Design review of the part shown in the three views and the two pictorial views. Dimensions are in mm from the part's minimum x, y and z. Round coordinates to 2 decimals unless told otherwise and drop trailing zeros. Loops run counter-clockwise (first coordinate to the right, second up) from the corner with the lowest first, then second, coordinate; pieces in that order, holes last. Notation, with made-up numbers: M 82,17.5 L 136,17.5 A24 ccw 136,52.5 Z; hole C 20,18 d10. An arc over 180 degrees is marked long. Answer as CSV lines item,"result". Start each with the question number.
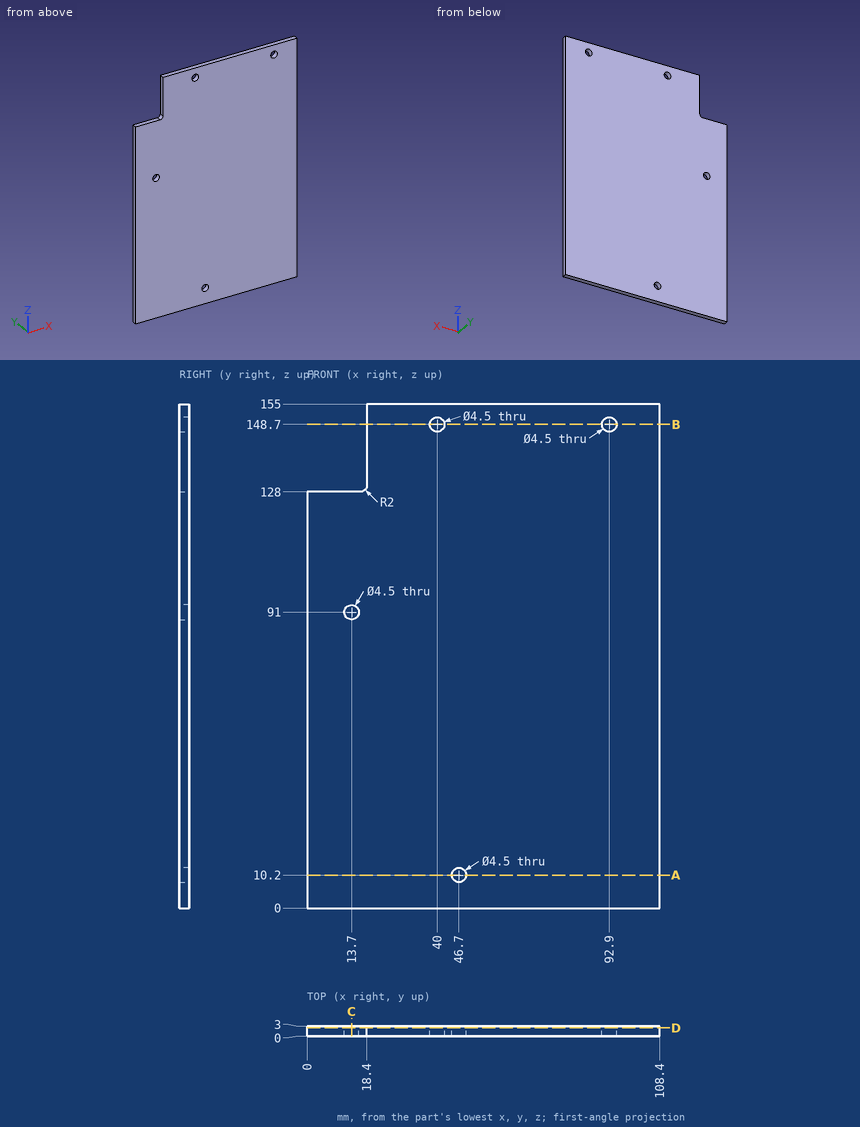
Item 1: Insertion check: pin 1 Ø0.9 at (x, y) = (10, 1) entering from +Z. The pin has a flat end and moves straight along its axis. Give the tip position at first contact, or say it passes through.
Item 2: To check wall thickness, follow line 1 (X direction, y = 1.75, z = 10.2); line 2 (Z direction, x = 15, y = 2.7); line 3 (X direction, y = 1.3, z = 93). State the ranges of each line that lie inside material, in increasing order.
Item 3: Consider section B-B, the plane z = 148.7. Write out the cut boundary in (x, y).
Item 4: Consider section D-D, the plane y = 2.5. Write out the cut boundary in (x, z).
Item 5: Consider section C-C, the plane x = 13.7. Write out the cut boundary in (y, z).
Item 6: Consider section A-A, the plane z = 10.2. Write out the cut boundary in (x, y), then the cut area to 3 significant figures.
Found:
1,pin 1,"stops at z = 128"
2,line 1,"x = 0 to 44.45, 48.95 to 108.4"
2,line 2,"z = 0 to 89.16, 92.84 to 128"
2,line 3,"x = 0 to 12.67, 14.73 to 108.4"
3,outline,"M 18.4,0 L 37.75,0 L 37.75,3 L 18.4,3 Z; M 42.25,0 L 90.65,0 L 90.65,3 L 42.25,3 Z; M 95.15,0 L 108.4,0 L 108.4,3 L 95.15,3 Z"
4,outline,"M 0,0 L 108.4,0 L 108.4,155 L 18.4,155 L 18.4,130 A2 cw 16.4,128 L 0,128 Z; hole C 13.7,91 d4.5; hole C 40,148.7 d4.5; hole C 46.7,10.2 d4.5; hole C 92.9,148.7 d4.5"
5,outline,"M 0,0 L 3,0 L 3,88.75 L 0,88.75 Z; M 0,93.25 L 3,93.25 L 3,128 L 0,128 Z"
6,outline,"M 0,0 L 44.45,0 L 44.45,3 L 0,3 Z; M 48.95,0 L 108.4,0 L 108.4,3 L 48.95,3 Z"
6,area,"312 mm^2"
